Geometry: see drawing. Coordinates: mm, zero at the bounding-box minimum. A direction names the side the tool comes from. Coordinates: 2 decimals unless noted, no trailing zeros. Loops run counter-clockwise (first coordinate to the right, second up) from the corner with the lowest first, then second, coordinate; pieces in that order, holes last. Notation, with made-up numbers: (89, 59) - (99, 59) arc R20 cw to (99, 72) - close; hole circle Ø4 at (8.25, -16). An arc over 180 degrees is marked (long way). Write item = value, one per line. Start each with the question number.
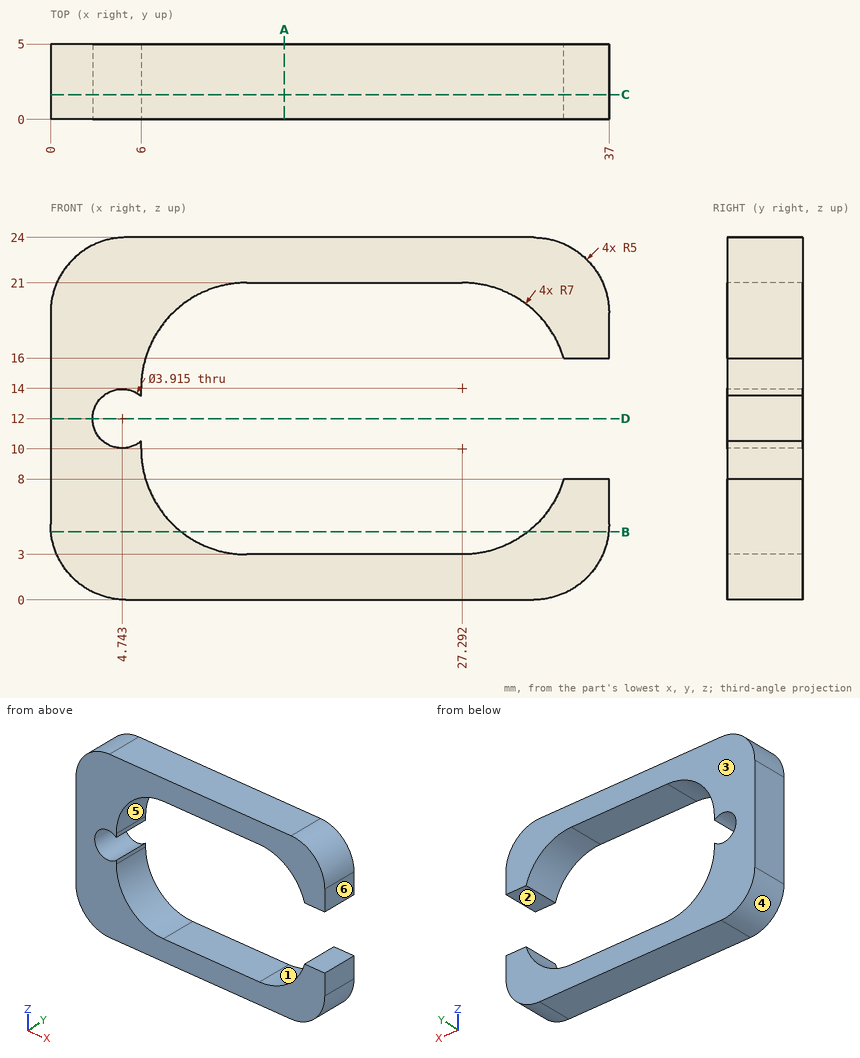
Item 1: Draft query along X for the marked faces 4, 5 and 6. Return one class per face: released by +X, released by -X, zero draft, split by the parting line, or undercut.
Item 2: Cut plane B-B (z = 4.5). Return the cut outline in (x, y) (1 decimal).
Item 3: Cut plane C-C (y = 1.65). Return the cut outline in (x, z) (1 decimal), then the cut area to 3 significant figures.
Item 4: Cut plane D-D (z = 12). Return the cut outline in (x, y) (1 decimal).
Item 5: Cut plane A-A (x = 15.5). Return the cut outline in (y, z), then the cut area to 3 significant figures.
Item 6: Reachability of the marked faces 1, 2 and 3 from +Z, -Z, +X, -X, +Y, -Y: full face, straight path, thin tool, end or side. Return the list, or none.
Item 7: First-contact query: pin 1 (1.5 mm diameter, centred on x = 22.5, y = 1.5, fed in from -Z); pin 2 (0.9 mm diameter, centred on x = 35.5, y = 2, fed in from +Z); pin 3 (2.5 mm diameter, centred on x = 35.5, y = 3, fed in from -Z) (1 decimal). Flat tips, straight axial feed; report the tip coordinate or a pass-through.
Item 8: Material intervals for L1, parallel to Z at x = 21, y = 3.35; L2, parallel to X at y = 2, z = 12 (1 decimal); L3, parallel to X at y = 0.6, z = 18.5 (1 decimal), sorted ascending. Write a range as [from, to].
Responses:
q1.face_4 = released by -X
q1.face_5 = undercut
q1.face_6 = released by +X
q2.outline = (0, 0) - (8.7, 0) - (8.7, 5) - (0, 5) - close; (31.6, 0) - (37, 0) - (37, 5) - (31.6, 5) - close
q3.outline = (0, 5) arc R5 ccw to (5, 0) - (32, 0) arc R5 ccw to (37, 5) - (37, 8) - (34, 8) arc R7 cw to (27.3, 3) - (13, 3) arc R7 cw to (6, 10) - (6, 10.5) arc R2 cw (long way) to (6, 13.5) - (6, 14) arc R7 cw to (13, 21) - (27.3, 21) arc R7 cw to (34, 16) - (37, 16) - (37, 19) arc R5 ccw to (32, 24) - (5, 24) arc R5 ccw to (0, 19) - close
q3.area = 367 mm2
q4.outline = (0, 0) - (2.8, 0) - (2.8, 5) - (0, 5) - close
q5.outline = (0, 0) - (5, 0) - (5, 3) - (0, 3) - close; (0, 21) - (5, 21) - (5, 24) - (0, 24) - close
q5.area = 30.0 mm2
q6.face_1 = +Y, -Y
q6.face_2 = +X, +Y, -Y
q6.face_3 = +Z, -Z, +X, -X, +Y
q7.pin_1 = 0
q7.pin_2 = 22.96
q7.pin_3 = 0.5
q8.L1 = [0, 3], [21, 24]
q8.L2 = [0, 2.8]
q8.L3 = [0, 7.6], [32.7, 37]
